```python
from build123d import *

# Parameters (mm, degrees)
F0_R     = 5
F1_DEPTH = 7
F2_R     = 1


with BuildPart() as f1:
    # F0 (on Top) → F1 (new body)
    with BuildSketch(Plane.XY):
        with BuildLine():
            ThreePointArc((21.3123029217, -1.9336765557), (14.7139218512, -1.3857264813), (9.5262793734, -5.5000001181))
            ThreePointArc((9.5262793734, -5.5000001181), (8.5570353366, -12.0497671944), (12.3307648053, -17.4901576816))
            ThreePointArc((12.3307648053, -17.4901576816), (21.5685847326, -17.9343458909), (26.3205080757, -10))
            ThreePointArc((26.3205080757, -10), (24.9666232205, -5.2526930589), (21.3123029217, -1.9336765557))
        make_face()
        with Locations((17.3205080757, -10)):
            Circle(F0_R, mode=Mode.SUBTRACT)
        with BuildLine():
            ThreePointArc((-8.3205080757, -10), (-8.6271756178, -7.6706286735), (-9.5262793594, -5.5000001424))
            ThreePointArc((-9.5262793594, -5.5000001424), (-14.7139219474, -1.3857264522), (-21.312303127, -1.9336766573))
            ThreePointArc((-21.312303127, -1.9336766573), (-25.1147367037, -14.5000000105), (-12.3307646513, -17.490157579))
            ThreePointArc((-12.3307646513, -17.490157579), (-9.3861621411, -14.2480765754), (-8.3205080757, -10))
        make_face()
        with Locations((-17.3205080757, -10)):
            Circle(F0_R, mode=Mode.SUBTRACT)
        with BuildLine():
            ThreePointArc((-9.5262793594, -5.5000001424), (-9.5262794827, 5.4999999288), (0, 11))
            ThreePointArc((0, 11), (-6.1568865898, 13.4354933529), (-8.9815384321, 19.4238338845))
            ThreePointArc((-8.9815384321, 19.4238338845), (-8.9473244085, 18.7122823092), (-8.9359158326, 18))
            ThreePointArc((-8.9359158326, 18), (-12.2816660211, 6.2683502062), (-21.312303127, -1.9336766573))
            ThreePointArc((-21.312303127, -1.9336766573), (-14.7139219474, -1.3857264522), (-9.5262793594, -5.5000001424))
        make_face()
        with BuildLine():
            ThreePointArc((12.3307648053, -17.4901576816), (8.5570353366, -12.0497671944), (9.5262793734, -5.5000001181))
            ThreePointArc((9.5262793734, -5.5000001181), (1.4e-08, -11), (-9.5262793594, -5.5000001424))
            ThreePointArc((-9.5262793594, -5.5000001424), (-8.6271756178, -7.6706286735), (-8.3205080757, -10))
            ThreePointArc((-8.3205080757, -10), (-9.3861621411, -14.2480765754), (-12.3307646513, -17.490157579))
            ThreePointArc((-12.3307646513, -17.490157579), (9.25e-08, -13.7590012964), (12.3307648053, -17.4901576816))
        make_face()
        with BuildLine():
            ThreePointArc((0, 11), (7.7781745931, 7.7781745931), (11, 0))
            ThreePointArc((11, 0), (10.6251840715, -2.847009562), (9.5262793734, -5.5000001181))
            ThreePointArc((9.5262793734, -5.5000001181), (14.7139218512, -1.3857264813), (21.3123029217, -1.9336765557))
            ThreePointArc((21.3123029217, -1.9336765557), (11.9156446994, 6.8795005684), (8.9815384291, 19.4238338374))
            ThreePointArc((8.9815384291, 19.4238338374), (6.1568865726, 13.4354933368), (0, 11))
        make_face()
        with BuildLine():
            ThreePointArc((-8.9815384321, 19.4238338845), (-6.1568865898, 13.4354933529), (0, 11))
            ThreePointArc((0, 11), (6.1568865726, 13.4354933368), (8.9815384291, 19.4238338374))
            ThreePointArc((8.9815384291, 19.4238338374), (8.9953834232, 19.7117690698), (9, 20))
            ThreePointArc((9, 20), (-0.2882309066, 28.995383424), (-8.9815384321, 19.4238338845))
        make_face()
        with Locations((0, 20)):
            Circle(F0_R, mode=Mode.SUBTRACT)
    extrude(amount=F1_DEPTH)

    # F2
    f2_edges = [f1.edges().sort_by_distance(p)[0] for p in [
        (-25.114737, -14.5, 7),
        (0, -13.759001, 7),
        (25.114737, -14.5, 7),
        (11.915645, 6.879501, 7),
        (-11.915645, 6.8795, 7),
        (0, 29, 7),
        (25.114737, -14.5, 0),
        (0, -13.759001, 0),
        (-25.114737, -14.5, 0),
        (-11.915645, 6.8795, 0),
        (0, 29, 0),
        (11.915645, 6.879501, 0),
    ]]
    fillet(f2_edges, radius=F2_R)


solid = f1.part
```
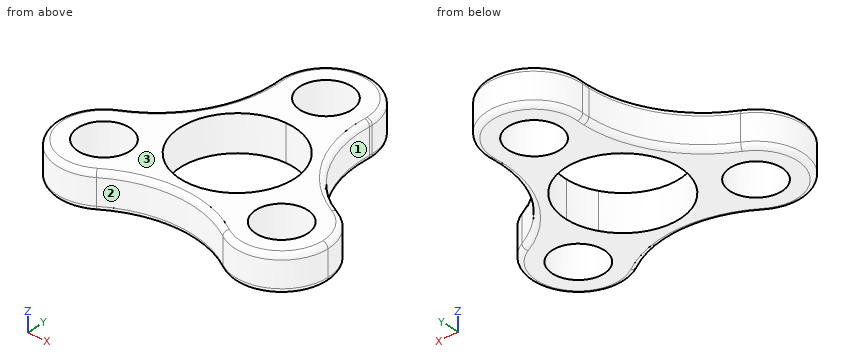
Geometry check sheet. Reference: the model listing, model coordinates, mm. Face numbers are marked on the shaded views. Coordinates: 2 decimals unless noted, no trailing zeros. Loops run counter-clockwise (first coordinate to the right, second up) from the corner with the lowest first, then second, coordinate; pieces in that order, holes last.
Item 1: Sectioned sample at A-A, the plane z = 4. Record the boundary of the cut face in (x, y).
Item 2: Go/stop test with flat-tipped pins: pin 1 Ø1 at (x, z) = (19, 5.5) entering from -Y; pin 2 Ø1.5 at (x, z) = (-9, 6) entering from +Y; pin 3 Ø1 at (y, z) = (-9.5, 6) entering from -X; pin 4 Ø3 at (y, z) = (8, 3) entering from +X. Record where each tip stops, or that it passes through.
Item 3: Release check for a two-part mould opening along X. For the marked faces 1, 2 and 3 record: released by +X, released by -X, zero draft, split by the parting line, or undercut.
Item 4: Thickness scan on line 1 (Y direction, x = 2, z = 1); line 2 (Y direction, x = 4, z = 1.5); line 3 (Y direction, x = -6, z = 5.5). Record the ranges inside material, lowest first.
Check result:
1. outline: (-21.31, -1.93) arc R9 ccw (long way) to (-12.33, -17.49) arc R22.24 cw to (12.33, -17.49) arc R9 ccw (long way) to (21.31, -1.93) arc R22.24 cw to (8.98, 19.42) arc R9 ccw (long way) to (-8.98, 19.42) arc R22.24 cw to start; hole circle Ø10 at (-17.32, -10); hole circle Ø22 at (0, 0); hole circle Ø10 at (0, 20); hole circle Ø10 at (17.32, -10)
2. pin 1: stops at y = -18.92
2. pin 2: stops at y = 23.6
2. pin 3: stops at x = -26.32
2. pin 4: stops at x = 12.14
3. face 1: released by +X
3. face 2: undercut
3. face 3: zero draft
4. line 1: y = -13.85 to -10.82, 10.82 to 15.42, 24.58 to 28.77
4. line 2: y = -14.12 to -10.25, 10.25 to 17, 23 to 28.06
4. line 3: y = -14.58 to -9.22, 9.22 to 26.71
